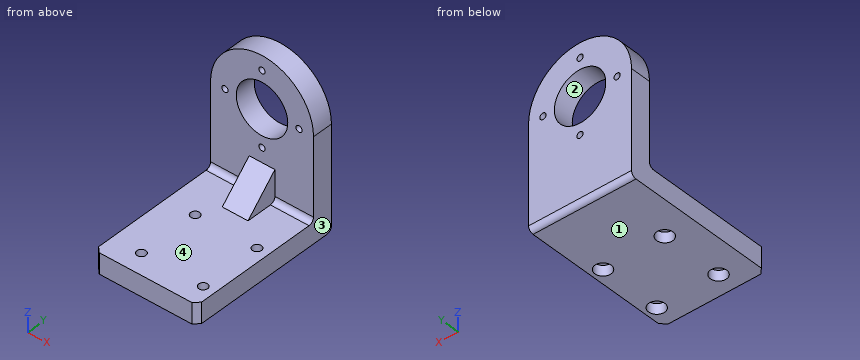
```python
from build123d import *

# Parameters (mm, degrees)
F0_W           = 200
F0_H           = 40
F0_R           = 7
F0_R_2         = 50
F1_DEPTH       = 40
F2_D           = 12.1
F3_DEPTH       = 300
F5_DEPTH       = 25
F7_SIZE        = 10
F8_R           = 10
F9_D           = 17.5
F9_CBORE_D     = 31.5
F9_CBORE_DEPTH = 20


with BuildPart() as f1:
    # F0 (on Front) → F1 (new body)
    with BuildSketch(Plane.XZ):
        with Locations((0, 20)):
            Rectangle(F0_W, F0_H)
        with BuildLine():
            Line((-100, 200), (-100, 40))
            Line((-100, 40), (100, 40))
            Line((100, 40), (100, 200))
            ThreePointArc((100, 200), (0, 300), (-100, 200))
        make_face()
        with Locations((0, 128)):
            Circle(F0_R, mode=Mode.SUBTRACT)
        with Locations((-72, 200)):
            Circle(F0_R, mode=Mode.SUBTRACT)
        with Locations((0, 200)):
            Circle(F0_R_2, mode=Mode.SUBTRACT)
        with Locations((72, 200)):
            Circle(F0_R, mode=Mode.SUBTRACT)
        with Locations((0, 272)):
            Circle(F0_R, mode=Mode.SUBTRACT)
        with Locations((-72, 200)):
            Circle(F0_R)
        with Locations((0, 272)):
            Circle(F0_R)
        with Locations((72, 200)):
            Circle(F0_R)
        with Locations((0, 128)):
            Circle(F0_R)
    extrude(amount=F1_DEPTH)

    # F2 (through all)
    with Locations(Plane(origin=(0, 0, 0), x_dir=(1, 0, 0), z_dir=(0, 1, 0))):
        with Locations((0, -272), (72, -200), (0, -128), (-72, -200)):
            Hole(F2_D / 2)

    # F0 (on Front) → F3 (join)
    with BuildSketch(Plane.XZ):
        with Locations((0, 20)):
            Rectangle(F0_W, F0_H)
    extrude(amount=F3_DEPTH)

    # F4 (on Right) → F5 (join, symmetric)
    with BuildSketch(Plane.YZ):
        Polygon((-100, 40), (-40, 40), (-40, 100), align=None)
    extrude(amount=F5_DEPTH, both=True)

    # F7
    f7_edges = [f1.edges().sort_by_distance(p)[0] for p in [
        (-100, -300, 20),
        (100, -300, 20),
    ]]
    chamfer(f7_edges, length=F7_SIZE)

    # F8
    f8_edges = [f1.edges().sort_by_distance(p)[0] for p in [
        (-62.5, -40, 40),
        (62.5, -40, 40),
        (0, 0, 0),
    ]]
    fillet(f8_edges, radius=F8_R)

    # F9 (through all)
    with Locations(Plane(origin=(0, 0, 0), x_dir=(1, 0, 0), z_dir=(0, 0, -1))):
        with Locations((-42.8080064058, 260), (77.1919935942, 260), (77.1919935942, 140), (-42.8080064058, 140)):
            CounterBoreHole(F9_D / 2, F9_CBORE_D / 2, F9_CBORE_DEPTH)


solid = f1.part
```
The listing builds one solid part. Answer for the finished solid, in the listing's coordinates (mm). Face numbers are marked on the shaded views. Coordinates: 2 decimals unless noted, no trailing zeros. Loops run counter-clockwise (first coordinate to the right, second up) from the corner with the lowest first, then second, coordinate; pieces in that order, holes last. Notation, with made-up numbers: (74, -24) -> (105, -24) arc R19 cw to (105, -7) -> close; hole circle Ø2 at (5.5, 50.25). An arc over 180 degrees is marked (long way). Return JSON: item names as keys, results as strings. Group by question number.
(1) A cutting plane is placed at D-D on z = 215.5. Write down the section's boundary in (x, y), and give its area (3 significant figures).
(2) Find the intervals of material crossed by probe 1 along X at (y, z) = (-260, 11); probe 2 along Z at (x, y) = (0, -27.5); probe 3 along X at (y, z) = (-140, 32), in increasing order. Write a range as from..to.
(3) Determine the mould class of the marked faces 1, 2, 3 and 4 for opening direction Z: released by +Z, released by -Z, zero draft, split by the parting line, or undercut.
(4) Given pin 1 Ø18 at (y, z) = (-64, 55) entering from +X; pin 2 Ø15.5 at (x, z) = (0, 128) entering from -Y; pin 3 Ø16 at (x, y) = (73, -138) entering from -Z; pin 4 Ø14 at (x, y) = (-42.81, -260) entering from +Z, each flat-ended and moving along its own axis, determine where each tip first touches the part or whether it passes through.
(5) A cutting plane is placed at C-C on y = -19. Write down the section's boundary in (x, z), and give its area (3 significant figures).
(6) A cutting plane is placed at B-B on x = 0. Write down the section's boundary in (y, z), and give its area (3 significant figures).
(7) A cutting plane is placed at A-A on y = -140. Write down the section's boundary in (x, z), and give its area (3 significant figures).
The answers:
{
 "1": {"outline": "(-98.79, -40) -> (-47.54, -40) -> (-47.54, 0) -> (-98.79, 0) -> close; (47.54, -40) -> (98.79, -40) -> (98.79, 0) -> (47.54, 0) -> close", "area": "4,100 mm^2"},
 "2": {"probe 1": "x = -100..-58.56, -27.06..61.44, 92.94..100", "probe 2": "z = 0..121.95, 134.05..150, 250..265.95, 278.05..300", "probe 3": "x = -100..-51.56, -34.06..68.44, 85.94..100"},
 "3": {"face 1": "released by -Z", "face 2": "undercut", "face 3": "zero draft", "face 4": "released by +Z"},
 "4": {"pin 1": "stops at x = 25", "pin 2": "stops at y = -40", "pin 3": "stops at z = 20", "pin 4": "passes through"},
 "5": {"outline": "(-100, 0) -> (100, 0) -> (100, 200) arc R100 ccw to (-100, 200) -> close; hole circle Ø12.1 at (-72, 200); hole circle Ø100 at (0, 200); hole circle Ø12.1 at (0, 128); hole circle Ø12.1 at (0, 272); hole circle Ø12.1 at (72, 200)", "area": "47,400 mm^2"},
 "6": {"outline": "(-300, 0) -> (-10, 0) arc R10 ccw to (0, 10) -> (0, 121.95) -> (-40, 121.95) -> (-40, 100) -> (-100, 40) -> (-300, 40) -> close; (-40, 134.05) -> (0, 134.05) -> (0, 150) -> (-40, 150) -> close; (-40, 250) -> (0, 250) -> (0, 265.95) -> (-40, 265.95) -> close; (-40, 278.05) -> (0, 278.05) -> (0, 300) -> (-40, 300) -> close", "area": "19,200 mm^2"},
 "7": {"outline": "(-100, 0) -> (-58.56, 0) -> (-58.56, 20) -> (-51.56, 20) -> (-51.56, 40) -> (-100, 40) -> close; (-34.06, 20) -> (-27.06, 20) -> (-27.06, 0) -> (61.44, 0) -> (61.44, 20) -> (68.44, 20) -> (68.44, 40) -> (-34.06, 40) -> close; (85.94, 20) -> (92.94, 20) -> (92.94, 0) -> (100, 0) -> (100, 40) -> (85.94, 40) -> close", "area": "6,040 mm^2"}
}
